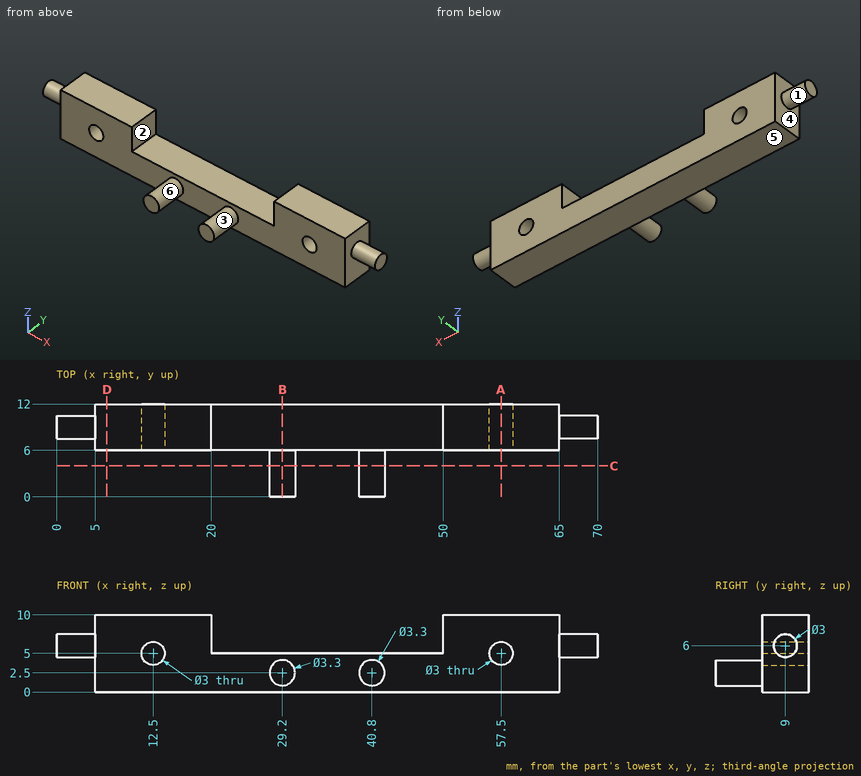
Verification items for this drawing (mm, ordinates from the low corner). A direction names the side the tool comes from. Round coordinates to 2 decimals unless told otherwise and drop trailing zeros. Loops run counter-clockwise (first coordinate to the right, second up) from the corner with the lowest first, then second, coordinate; pieces in that order, holes last. Notation, with made-up numbers: (68.5, 21.5) -> (112.5, 21.5) arc R7 ccw to (112.5, 30.5) -> close; hole circle Ø9 at (65.25, 76). An arc over 180 degrees is marked (long way). Answer in a Markdown table with one row per item.
Q1. Sectioned sample at D-D on x = 6.5. Enter the section's corners in (y, z).
Data:
| item | result |
|---|---|
| outline | (6, 0) -> (12, 0) -> (12, 10) -> (6, 10) -> close |
Q2. Sectioned sample at C-C on y = 4. Enter the section's corners in (x, z).
Data:
| item | result |
|---|---|
| outline | circle Ø3.3 at (29.2, 2.5); circle Ø3.3 at (40.8, 2.5) |
Q3. Go/stop test with flat-tipped pins: P1, Ø5, axis at y = 10.5, z = 6, coming from the -X side; P2, Ø1.5, axis at y = 7.5, z = 8, coming from the +X side; P3, Ø4, axis at x = 53.5, z = 8, coming from the -Y side; P4, Ø6.5, axis at x = 38, y = 10, coming from the +Z side. Record where each tip stops, or that it passes through.
Data:
| item | result |
|---|---|
| P1 | stops at x = 0 |
| P2 | stops at x = 65 |
| P3 | stops at y = 6 |
| P4 | stops at z = 5 |
Q4. Sectioned sample at A-A on x = 57.5. Enter the section's corners in (y, z).
Data:
| item | result |
|---|---|
| outline | (6, 0) -> (12, 0) -> (12, 3.5) -> (6, 3.5) -> close; (6, 6.5) -> (12, 6.5) -> (12, 10) -> (6, 10) -> close |
Q5. Release check for a two-part mould opening along X. For the marked faces 4, 5 and 6 record: released by +X, released by -X, zero draft, split by the parting line, or undercut.
Data:
| item | result |
|---|---|
| face 4 | released by -X |
| face 5 | zero draft |
| face 6 | undercut |
Q6. Set-up check for the marked faces 1, 2 and 3: record each of +Z, -Z, +X, -X, +Y, -Y from which the full face is reachable in a straight line by a thin tool's end or side.
Data:
| item | result |
|---|---|
| face 1 | -X |
| face 2 | +Z, +Y, -Y |
| face 3 | -Y |
Q7. Sectioned sample at B-B on x = 29.2. Enter the section's corners in (y, z).
Data:
| item | result |
|---|---|
| outline | (0, 0.85) -> (6, 0.85) -> (6, 0) -> (12, 0) -> (12, 5) -> (6, 5) -> (6, 4.15) -> (0, 4.15) -> close |
Q8. Thickness scan on L1, parallel to Z at x = 12.5, y = 10.3; L2, parallel to Y at x = 20.5, z = 4; L3, parallel to X at y = 6.75, z = 1.5. Record the ranges inside material, lowest first.
Data:
| item | result |
|---|---|
| L1 | z = 0 to 3.5, 6.5 to 10 |
| L2 | y = 6 to 12 |
| L3 | x = 5 to 65 |
